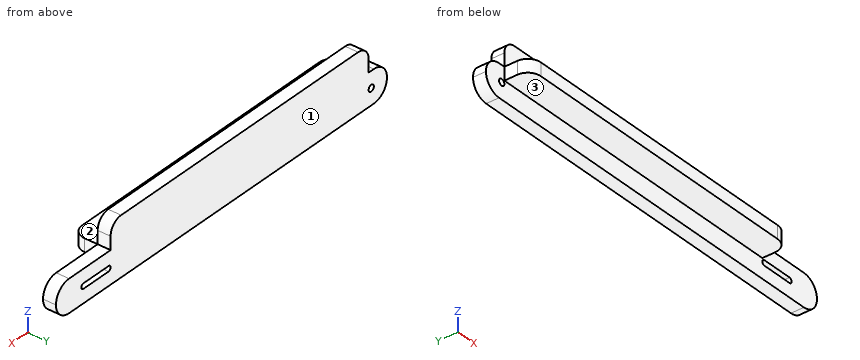
from build123d import *

# Parameters (mm, degrees)
F0_W     = 315
F0_H     = 25
F0_R     = 2.5
F1_DEPTH = 10
F2_R     = 12.49999
F3_W     = 245.5
F3_H     = 10
F4_DEPTH = 20
F5_W     = 245.5
F5_H     = 10
F6_DEPTH = 20
F7_R     = 10
F8_R     = 10


# Not quite as in the source:
# - a fillet or chamfer is up to 0.001 mm smaller than in the source, because OpenCascade refuses the exact size


with BuildPart() as f1:
    # F0 (on Front) → F1 (new body)
    with BuildSketch(Plane.XZ):
        with Locations((167.5, 12.5)):
            Rectangle(F0_W, F0_H)
        with Locations((25, 12.5)):
            Circle(F0_R, mode=Mode.SUBTRACT)
        with BuildLine():
            ThreePointArc((298.861, 14.5), (300.861, 12.5), (298.861, 10.5))
            Line((298.861, 10.5), (275, 10.5))
            ThreePointArc((275, 10.5), (273, 12.5), (275, 14.5))
            Line((275, 14.5), (298.861, 14.5))
        make_face(mode=Mode.SUBTRACT)
    extrude(amount=F1_DEPTH)

    # F2 (radius 12.5 in the source; OpenCascade refuses exactly that, so slightly less here)
    f2_edges = [f1.edges().sort_by_distance(p)[0] for p in [
        (10, -5, 25),
        (10, -5, 0),
        (325, -5, 0),
        (325, -5, 25),
    ]]
    fillet(f2_edges, radius=F2_R)

    # F3 (on face) → F4 (join)
    with BuildSketch(Plane.XZ.offset(10)):
        with Locations((150.25, 20)):
            Rectangle(F3_W, F3_H)
    extrude(amount=F4_DEPTH)

    # F5 (on face) → F6 (join)
    with BuildSketch(Plane.XY.offset(25)):
        with Locations((150.25, -5)):
            Rectangle(F5_W, F5_H)
    extrude(amount=F6_DEPTH)

    # F7
    f7_edges = [f1.edges().sort_by_distance(p)[0] for p in [
        (27.5, -5, 45),
    ]]
    fillet(f7_edges, radius=F7_R)

    # F8
    f8_edges = [f1.edges().sort_by_distance(p)[0] for p in [
        (273, -5, 45),
        (273, -30, 20),
        (27.5, -30, 20),
    ]]
    fillet(f8_edges, radius=F8_R)


solid = f1.part
Verification items for the finished model (mm, model axes). Face numbers are marked on the shaded views. A direction names the side the tool comes from. Coordinates: 2 decimals unless noted, no trailing zeros. Order: outer loops, then holes, each group sorted by start corner. A loop starts at its lowest first (then second) coordinate and runs counter-clockwise, first axis right, second up. Notation, with made-up numbers: (17, -21) -> (36, -21) arc R19 cw to (36, -7) -> close; hole circle Ø5 at (71.5, 53). An arc over 180 degrees is marked (long way). Put each result on its own line as item: value. Start each with the question number.
1. Material ranges on L1, parallel to Z at x = 25, y = -6; L2, parallel to Z at x = 268, y = -18.5; L3, parallel to Y at x = 107.5, z = 3.5, recorded low to high. Write a range as [from, to].
2. Access from +Z, -Z, +X, -X, +Y, -Y to the whole of each face (thin tool, end or side, straight path). Record for the marked faces 1, 2 and 3.
3. Cross-section at C-C, the plane z = 41.5. Record the boundary of the cut face in (x, y).
4. Go/stop test with flat-tipped pins: pin 1 Ø12 at (x, z) = (185.5, 37.5) entering from -Y; pin 2 Ø4 at (y, z) = (-5, 31.5) entering from -X; pin 3 Ø6 at (x, y) = (188, -16.5) entering from -Z; pin 4 Ø4 at (x, z) = (25, 12.5) entering from +Y. Record where each tip stops, or that it passes through.
5. Cross-section at D-D, the plane y = -25.5. Record the boundary of the cut face in (x, z).
6. Cross-section at B-B, the plane x = 257.5. Record the boundary of the cut face in (y, z).
7. Cross-section at A-A, the plane y = -4.75. Count the separate pieces of the cut face and the enclosed holes in it, then the cut area to 3 significant figures.
Computed:
1. L1: [0, 10], [15, 25]
1. L2: [15, 25]
1. L3: [-10, 0]
2. face 1: +Z, -Z, +X, -X, +Y
2. face 2: +Z, +X, -X, -Y
2. face 3: -Z, +X, -X, -Y
3. outline: (29.9, -10) -> (270.6, -10) -> (270.6, 0) -> (29.9, 0) -> close
4. pin 1: y = -10
4. pin 2: x = 27.5
4. pin 3: z = 15
4. pin 4: through
5. outline: (29.15, 15) -> (271.35, 15) -> (271.35, 25) -> (29.15, 25) -> close
6. outline: (-30, 15) -> (-10, 15) -> (-10, 0) -> (0, 0) -> (0, 45) -> (-10, 45) -> (-10, 25) -> (-30, 25) -> close
7. separate pieces: 1
7. enclosed holes: 2
7. area: 12,500 mm2
